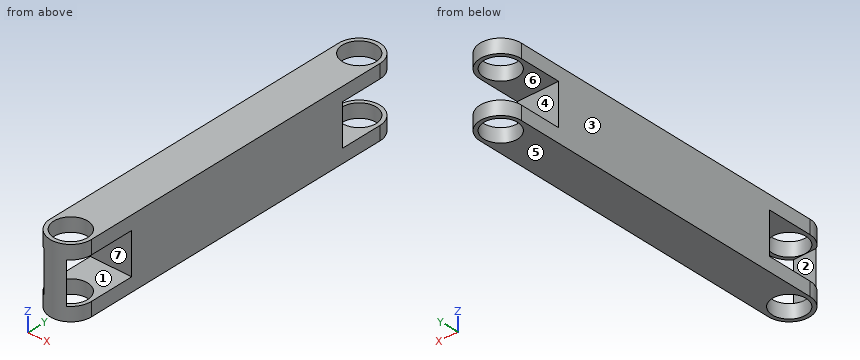
```python
from build123d import *

# Parameters (mm, degrees)
ESTRUSIONE_ESTRUSIONE1_DEPTH      = 5
ESTRUSIONE_ESTRUSIONE1_DEPTH_BACK = 5
SCHIZZO1_R                        = 2.45
TAGLIO_ESTRUSIONE1_DEPTH          = 50.921702695
TAGLIO_ESTRUSIONE1_DEPTH_BACK     = 50.921702695
SCHIZZO2_W                        = 6
SCHIZZO2_H                        = 9


with BuildPart() as part:
    # Schizzo1 → Estrusione-Estrusione1 (new, two sides: drawn at the far end of the back side and taken through both)
    with BuildSketch(Plane.XY.offset(-ESTRUSIONE_ESTRUSIONE1_DEPTH_BACK)):
        with BuildLine():
            Line((-3, 0), (-3, 46.58))
            ThreePointArc((-3, 46.58), (0, 49.58), (3, 46.58))
            Line((3, 46.58), (3, 0))
            ThreePointArc((3, 0), (0, -3), (-3, 0))
        make_face()
        Circle(SCHIZZO1_R, mode=Mode.SUBTRACT)
        with Locations((0, 46.58)):
            Circle(SCHIZZO1_R, mode=Mode.SUBTRACT)
    extrude(amount=ESTRUSIONE_ESTRUSIONE1_DEPTH + ESTRUSIONE_ESTRUSIONE1_DEPTH_BACK)

    # Schizzo2 → Taglio-Estrusione1 (cut, two sides: drawn at the far end of the back side and taken through both)
    with BuildSketch(Plane(origin=(0, 0, 0), x_dir=(0, 0, -1), z_dir=(1, 0, 0)).offset(-TAGLIO_ESTRUSIONE1_DEPTH_BACK)):
        with Locations((0, 45.08)):
            Rectangle(SCHIZZO2_W, SCHIZZO2_H)
        with Locations((0, 2)):
            Rectangle(SCHIZZO2_W, SCHIZZO2_H)
    extrude(amount=TAGLIO_ESTRUSIONE1_DEPTH + TAGLIO_ESTRUSIONE1_DEPTH_BACK, mode=Mode.SUBTRACT)


solid = part.part
```
Work out the finished part from the listing and answer in its coordinate system (mm). Face numbers are marked on the shaded views. A direction names the side the tool comes from. Round coordinates to 2 decimals unless told otherwise and drop trailing zeros. Order: outer loops, then holes, each group sorted by start corner. A loop starts at its lowest first (then second) coordinate and runs counter-clockwise, first axis right, second up.
Q1. Given pin 1 Ø1 at (x, z) = (1.5, 0) entering from +Y, flat-ended and moving along its own axis, determine where the tip first touches the part or whether it passes through.
Solution:
pin 1: stops at y = 40.58
Q2. A tool of negligible diameter and unlimited length cuts with its end or side. For the marked faces 5, 6 and 7, from which of +Z, -Z, +X, -X, +Y, -Y can it reach the whole face along a straight path? Write none if from no direction.
Solution:
face 5: -Z, +X, -X, +Y, -Y
face 6: +X, -X, +Y
face 7: +X, -X
Q3. A cutting plane is placed at B-B, the plane y = 3.5. Determine the outline of the cut face in (x, z), then the cut area to 3 significant figures.
Solution:
outline: (-3, -5) - (3, -5) - (3, -3) - (-3, -3) - close; (-3, 3) - (3, 3) - (3, 5) - (-3, 5) - close
area: 24.0 mm2
Q4. A cutting plane is placed at D-D, the plane y = 45. Determine the outline of the cut face in (x, z).
Solution:
outline: (-3, -5) - (-1.87, -5) - (-1.87, -3) - (-3, -3) - close; (-3, 3) - (-1.87, 3) - (-1.87, 5) - (-3, 5) - close; (1.87, -5) - (3, -5) - (3, -3) - (1.87, -3) - close; (1.87, 3) - (3, 3) - (3, 5) - (1.87, 5) - close
Q5. A cutting plane is placed at C-C, the plane z = 3.5. Determine the outline of the cut face in (x, y).
Solution:
outline: (-3, 0) arc R3 ccw to (3, 0) - (3, 46.58) arc R3 ccw to (-3, 46.58) - close; hole circle Ø4.9 at (0, 0); hole circle Ø4.9 at (0, 46.58)
Q6. The mould has two halves that part along Y. Classify the marked faces 1, 2, 3 and 4: pulls with the +Y half, pulls with the -Y half, needs draft (parallel to the pull), parting line crosses it, or undercut.
Solution:
face 1: undercut
face 2: undercut
face 3: needs draft
face 4: pulls with the +Y half
Q7. A cutting plane is placed at A-A, the plane x = 0. Determine the outline of the cut face in (y, z).
Solution:
outline: (-3, -5) - (-2.45, -5) - (-2.45, -3) - (-2.5, -3) - (-2.5, 3) - (-2.45, 3) - (-2.45, 5) - (-3, 5) - close; (2.45, -5) - (44.13, -5) - (44.13, -3) - (40.58, -3) - (40.58, 3) - (44.13, 3) - (44.13, 5) - (2.45, 5) - (2.45, 3) - (6.5, 3) - (6.5, -3) - (2.45, -3) - close; (49.03, -5) - (49.58, -5) - (49.58, -3) - (49.03, -3) - close; (49.03, 3) - (49.58, 3) - (49.58, 5) - (49.03, 5) - close
Q8. Find the intervals of material crossed by line 1 along Y through (x, z) = (0, -3.9); line 2 along X through (y, z) = (0, 4.2); line 3 along Z through (x, y) = (2.75, 1), in increasing order.
Solution:
line 1: y = -3 to -2.45, 2.45 to 44.13, 49.03 to 49.58
line 2: x = -3 to -2.45, 2.45 to 3
line 3: z = -5 to -3, 3 to 5
